```python
from build123d import *

# Parameters (mm, degrees)
SKETCH1_W           = 152.4
SKETCH1_H           = 50
BOSS_EXTRUDE1_DEPTH = 6.35
CUT_EXTRUDE2_REACH  = 82.447
SKETCH3_R           = 3.429


with BuildPart() as part:
    # Sketch1 → Boss-Extrude1 (new body)
    with BuildSketch(Plane(origin=(0, 0, 0), x_dir=(1, 0, 0), z_dir=(0, 1, 0))):
        Rectangle(SKETCH1_W, SKETCH1_H)
    extrude(amount=BOSS_EXTRUDE1_DEPTH)

    # Sketch3 → Cut-Extrude2 (cut, up to next)
    with BuildSketch(Plane.XZ, mode=Mode.PRIVATE) as cut_extrude2_sk1:
        with Locations(Location((-63.5, 12.3, 0), (0, 0, 270))):
            Circle(SKETCH3_R)
    cut_extrude2_tool1 = extrude(cut_extrude2_sk1.sketch, amount=-CUT_EXTRUDE2_REACH, mode=Mode.PRIVATE) & part.part
    # Sketch3 → Cut-Extrude2 (cut, up to next)
    with BuildSketch(Plane.XZ, mode=Mode.PRIVATE) as cut_extrude2_sk2:
        with Locations(Location((-63.5, -12.3, 0), (0, 0, 90))):
            Circle(SKETCH3_R)
    cut_extrude2_tool2 = extrude(cut_extrude2_sk2.sketch, amount=-CUT_EXTRUDE2_REACH, mode=Mode.PRIVATE) & part.part
    # Sketch3 → Cut-Extrude2 (cut, up to next)
    with BuildSketch(Plane.XZ, mode=Mode.PRIVATE) as cut_extrude2_sk3:
        with Locations(Location((63.5, 12.3, 0), (0, 0, 90))):
            Circle(SKETCH3_R)
    cut_extrude2_tool3 = extrude(cut_extrude2_sk3.sketch, amount=-CUT_EXTRUDE2_REACH, mode=Mode.PRIVATE) & part.part
    # Sketch3 → Cut-Extrude2 (cut, up to next)
    with BuildSketch(Plane.XZ, mode=Mode.PRIVATE) as cut_extrude2_sk4:
        with Locations(Location((63.5, -12.3, 0), (0, 0, 270))):
            Circle(SKETCH3_R)
    cut_extrude2_tool4 = extrude(cut_extrude2_sk4.sketch, amount=-CUT_EXTRUDE2_REACH, mode=Mode.PRIVATE) & part.part
    # Sketch3 → Cut-Extrude2 (cut, up to next)
    with BuildSketch(Plane.XZ, mode=Mode.PRIVATE) as cut_extrude2_sk5:
        with Locations(Location((-12.698950153, 12.699994489, 0), (0, 0, 270))):
            Circle(SKETCH3_R)
    cut_extrude2_tool5 = extrude(cut_extrude2_sk5.sketch, amount=-CUT_EXTRUDE2_REACH, mode=Mode.PRIVATE) & part.part
    # Sketch3 → Cut-Extrude2 (cut, up to next)
    with BuildSketch(Plane.XZ, mode=Mode.PRIVATE) as cut_extrude2_sk6:
        with Locations(Location((-12.698950153, -12.699994489, 0), (0, 0, 270))):
            Circle(SKETCH3_R)
    cut_extrude2_tool6 = extrude(cut_extrude2_sk6.sketch, amount=-CUT_EXTRUDE2_REACH, mode=Mode.PRIVATE) & part.part
    add(cut_extrude2_tool1.solids().sort_by_distance((-63.5, 0, 12.3))[0], mode=Mode.SUBTRACT)
    add(cut_extrude2_tool2.solids().sort_by_distance((-63.5, 0, -12.3))[0], mode=Mode.SUBTRACT)
    add(cut_extrude2_tool3.solids().sort_by_distance((63.5, 0, 12.3))[0], mode=Mode.SUBTRACT)
    add(cut_extrude2_tool4.solids().sort_by_distance((63.5, 0, -12.3))[0], mode=Mode.SUBTRACT)
    add(cut_extrude2_tool5.solids().sort_by_distance((-12.69895, 0, 12.699994))[0], mode=Mode.SUBTRACT)
    add(cut_extrude2_tool6.solids().sort_by_distance((-12.69895, 0, -12.699994))[0], mode=Mode.SUBTRACT)


solid = part.part
```
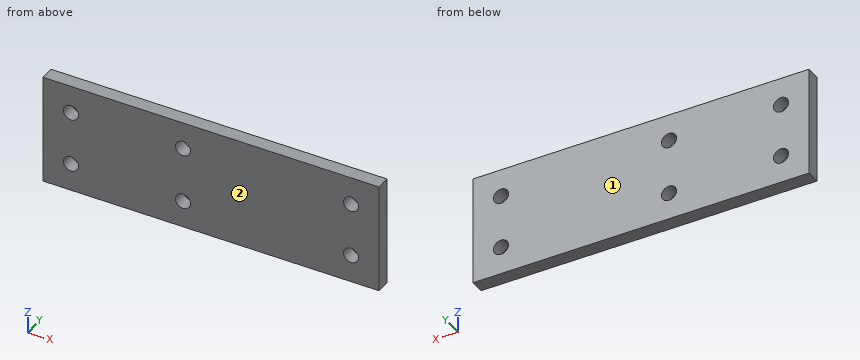
For this review, take the finished solid that the model builds, in its own axes (mm). Face numbers are marked on the shaded views. Coordinates: 2 decimals unless noted, no trailing zeros. Write each loop counter-clockwise with the first axis right and the second up, starting at its lowest first coordinate (ties: lowest second). Pieces come first, ordered by that corner, then holes. Notation, with made-up numbers: (39, -19) -> (61, -19) arc R32 cw to (61, 11) -> close; hole circle Ø8 at (-16, 45). An arc over 180 degrees is marked (long way). Put each result on its own line as item: value.
Q1. Wall thickness on L1, parallel to X at y = 2.5, z = -12.3; L2, parallel to Z at x = -62.5, y = 3.5; L3, parallel to X at y = 5, z = -14: over which ranges is each line inside the solid? List them lowest first.
From the geometry:
L1: x = -76.2 to -66.93, -60.07 to -16.1, -9.29 to 60.07, 66.93 to 76.2
L2: z = -25 to -15.58, -9.02 to 9.02, 15.58 to 25
L3: x = -76.2 to -66.48, -60.52 to -15.87, -9.53 to 60.52, 66.48 to 76.2
Q2. The part is to be moulded in two halves that separate along Y. For the marked faces 1 and 2, say which applies: +Y half, -Y half, draft (parallel to the pull), parting line (faces both ways), or undercut.
From the geometry:
face 1: +Y half
face 2: -Y half
Q3. Take a section at A-A, the plane x = -63.5. State the section outline as (y, z) points, then the cut area to 3 significant figures.
From the geometry:
outline: (0, -25) -> (6.35, -25) -> (6.35, -15.73) -> (0, -15.73) -> close; (0, -8.87) -> (6.35, -8.87) -> (6.35, 8.87) -> (0, 8.87) -> close; (0, 15.73) -> (6.35, 15.73) -> (6.35, 25) -> (0, 25) -> close
area: 230 mm2
Q4. Clearance check with a flat-ended pin moving along its axis: pin 1 Ø5.5 at (x, z) = (63.5, 12.3) entering from +Y. State where the tip first meets the part, or that it passes through.
From the geometry:
pin 1: passes through
Q5. Take a section at B-B, the plane z = -12.3. State the section outline as (x, y) points.
From the geometry:
outline: (-76.2, 0) -> (-66.93, 0) -> (-66.93, 6.35) -> (-76.2, 6.35) -> close; (-60.07, 0) -> (-16.1, 0) -> (-16.1, 6.35) -> (-60.07, 6.35) -> close; (-9.29, 0) -> (60.07, 0) -> (60.07, 6.35) -> (-9.29, 6.35) -> close; (66.93, 0) -> (76.2, 0) -> (76.2, 6.35) -> (66.93, 6.35) -> close
Q6. Take a section at C-C, the plane y = 2.25. State the section outline as (x, z) points.
From the geometry:
outline: (-76.2, -25) -> (76.2, -25) -> (76.2, 25) -> (-76.2, 25) -> close; hole circle Ø6.86 at (-63.5, -12.3); hole circle Ø6.86 at (-63.5, 12.3); hole circle Ø6.86 at (-12.7, -12.7); hole circle Ø6.86 at (-12.7, 12.7); hole circle Ø6.86 at (63.5, -12.3); hole circle Ø6.86 at (63.5, 12.3)
